Autodesk Inventor part; units mm, degrees
ref_plane "YZ Plane" through (0, 0, 0) normal (1, 0, 0) x (0, 1, 0)
ref_plane "XZ Plane" through (0, 0, 0) normal (0, 1, 0) x (-1, 0, 0)
ref_plane "XY Plane" through (0, 0, 0) normal (0, 0, 1) x (1, 0, 0)
sketch "Szkic1" plane through (0, 0, 0) normal (0, 1, 0) x (-1, 0, 0)
  circle A0 centre (0, 0) radius 15
  circle A1 centre (0, 0) radius 8.25
  circle A2 centre (0, 0) radius 12.5
  dimension "d0" = 30
  dimension "d1" = 16.5
  dimension "d2" = 25
extrude "Wyciągnięcie proste1" add sketch "Szkic1" along normal blind 17 contours A0 | A1 | A2
extrude "Wyciągnięcie proste2" cut sketch "Szkic1" against normal blind 35 from surface at 17 contours A1
extrude "Wyciągnięcie proste3" cut sketch "Szkic1" along normal blind 7 contours A0
chamfer "Faza1" distance 1 angle 45 2 edges at (12.5, 0, 0) (8.25, 17, 0)
properties part number "X_end_floating_cup" material "Tworzywo sztuczne ABS"
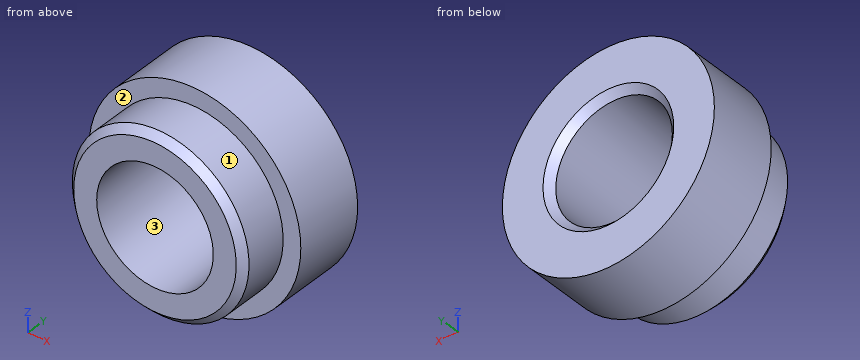
Source: CAD feature listing. Evaluate the final solid. Frame: model axes, mm. Face numbers are marked on the shaded views. Round coordinates to 2 decimals unless told otherwise and drop trailing zeros. Loops run counter-clockwise (first coordinate to the right, second up) from the corner with the lowest first, then second, coordinate; pieces in that order, holes last. Notation, with made-up numbers: M 34,72.25 L 75,72.25 A10 cw 75,87.25 Z; hole C 28,68 d4. An arc over 180 degrees is marked long. Use a Markdown table: item, result. Add a question column.
1. Section query C-C on y = 3.5. Return the cut outline in (x, z).
2. Mould query, pull axis Z, two halves, no side actions, for the marked faces 1, 2 and 3. Classes: pulls with the +Z half, pulls with the -Z half, needs draft (parallel to the pull), parting line crosses it, or undercut.
3. Section query D-D on y = 7.75. Return the cut outline in (x, z).
4. Section query B-B on z = 0. Return the cut outline in (x, y), then the cut area to 4 significant figures.
5. Section query A-A on x = 0. Return the cut outline in (y, z).
6. Line query: line 1 (Z direction, x = 0, y = 12.5); line 2 (Z direction, x = 0, y = 5.5); line 3 (X direction, y = 13, z = 1). Output: solid intervals per line, ascending.
7. Contact query for flat-ended pins moving along their axis: P1, Ø8, axis at x = -6, y = 11, coming from the -Z side; P2, Ø10, axis at x = 7.5, y = 10.5, coming from the +Z side; P3, Ø2, axis at x = -6.5, z = -11.5, coming from the -Y side. Output: stop coordinate, or through.
Reported:
| question | item | result |
|---|---|---|
| 1 | outline | C 0,0 d25; hole C 0,0 d16.5 |
| 2 | face 1 | parting line crosses it |
| 2 | face 2 | needs draft |
| 2 | face 3 | undercut |
| 3 | outline | C 0,0 d30; hole C 0,0 d16.5 |
| 4 | outline | M -15,7 L -12.5,7 L -12.5,1 L -11.5,0 L -8.25,0 L -8.25,16 L -9.25,17 L -15,17 Z; M 8.25,0 L 11.5,0 L 12.5,1 L 12.5,7 L 15,7 L 15,17 L 9.25,17 L 8.25,16 Z |
| 4 | area | 192.5 mm² |
| 5 | outline | M 0,-11.5 L 1,-12.5 L 7,-12.5 L 7,-15 L 17,-15 L 17,-9.25 L 16,-8.25 L 0,-8.25 Z; M 0,8.25 L 16,8.25 L 17,9.25 L 17,15 L 7,15 L 7,12.5 L 1,12.5 L 0,11.5 Z |
| 6 | line 1 | z = -15 to -8.25, 8.25 to 15 |
| 6 | line 2 | z = -12.5 to -8.25, 8.25 to 12.5 |
| 6 | line 3 | x = -14.97 to -8.19, 8.19 to 14.97 |
| 7 | P1 | stops at z = -14.87 |
| 7 | P2 | stops at z = 14.79 |
| 7 | P3 | stops at y = 0.71 |
